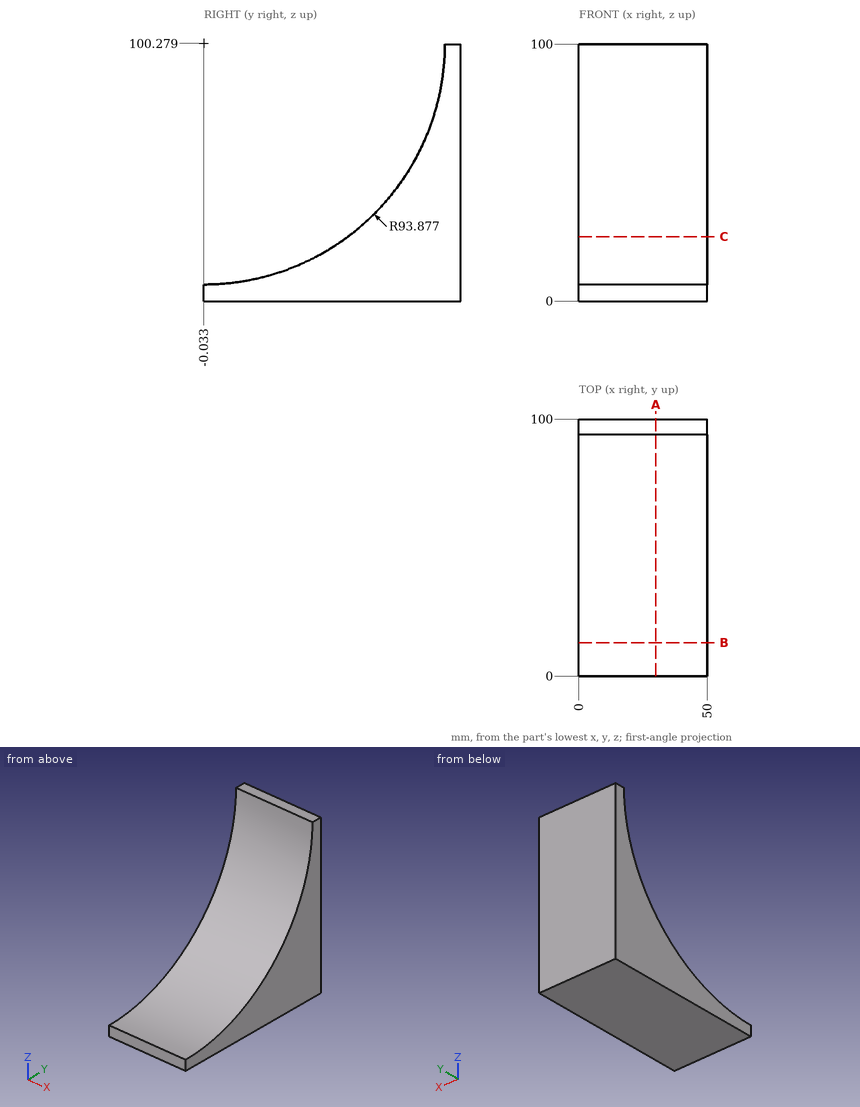
Geometry: see drawing. Coordinates: mm, zero at the bounding-box minimum. Coordinates: 2 decimals unless noted, no trailing zeros. Write each loop counter-clockwise with the first axis right and the second up, starting at its lowest first coordinate (ties: lowest second). Pieces come first, ordered by that corner, then holes.
1) Material intervals for line 1 along Z through (x, y) = (24.5, 40) (1 decimal); line 2 along Y through (x, z) = (8, 17) (1 decimal); line 3 along Y through (x, z) = (25.5, 24), sorted ascending.
2) Section C-C on z = 25. Output: boundary loops of the cut face in (x, y).
3) Section A-A on x = 30. Output: boundary loops of the cut face in (y, z), and give its area (3 significant figures).
4) Section B-B on y = 13. Output: boundary loops of the cut face in (x, z).
5) Pin query (flat end, axial travel): pin 1 Ø4 at (x, y) = (12.5, 69) entering from +Z; pin 2 Ø2 at (x, z) = (13, 59) entering from -Y (1 decimal); pin 3 Ø5 at (x, z) = (29.5, 51.5) entering from -Y. Return the tip coordinate at first contact, or that it passes through.
Check result:
1. line 1: z = 0 to 15.4
1. line 2: y = 43.3 to 100
1. line 3: y = 54.69 to 100
2. outline: (0, 56.06) - (50, 56.06) - (50, 100) - (0, 100) - close
3. outline: (0, 0) - (100, 0) - (100, 100) - (93.84, 100) arc R93.88 cw to (0, 6.4) - close
3. area: 3,110 mm2
4. outline: (0, 0) - (50, 0) - (50, 7.31) - (0, 7.31) - close
5. pin 1: stops at z = 38.9
5. pin 2: stops at y = 83.8
5. pin 3: stops at y = 78.6
